Autodesk Inventor part; units mm, degrees
ref_plane "YZ Plane" through (0, 0, 0) normal (1, 0, 0) x (0, 1, 0)
ref_plane "XZ Plane" through (0, 0, 0) normal (0, 1, 0) x (-1, 0, 0)
ref_plane "XY Plane" through (0, 0, 0) normal (0, 0, 1) x (1, 0, 0)
sketch "スケッチ1" plane through (0, 0, 0) normal (0, 0, 1) x (1, 0, 0)
  circle A0 centre (0, 0) radius 23.5
  circle A1 centre (0, 0) radius 4
  dimension "d0" = 47
  dimension "d1" = 8
extrude "押し出し1" add sketch "スケッチ1" along normal blind 2
sketch "スケッチ2" plane through (0, 0, 2) normal (0, 0, 1) x (1, 0, 0)
  circle A0 centre (0, 0) radius 6.5 construction
  circle A1 centre (-6.5, 0) radius 1.75
  circle A2 centre (6.5, 0) radius 1.75
  dimension "d4" = 13
  dimension "d5" = 3.5
extrude "押し出し2" cut sketch "スケッチ2" against normal blind 2
chamfer "面取り1" distance 1.6 angle 45 2 edges at (-8.25, 0, 2) (4.75, 0, 2)
properties part number "SlitDiscSupport1"
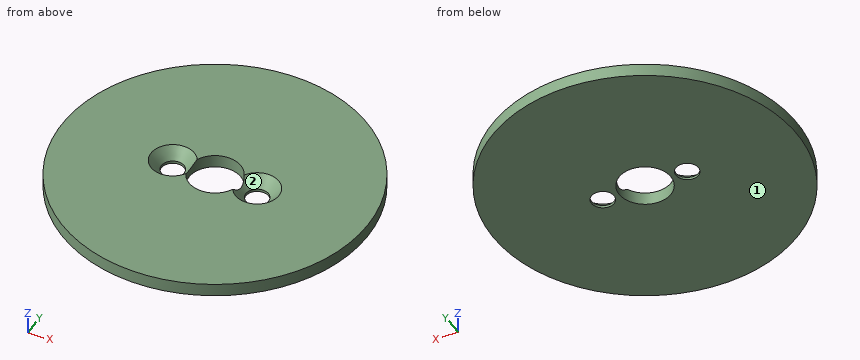
Part model, mm, in its own coordinate system. Face numbers are marked on the shaded views. Round coordinates to 2 decimals unless told otherwise and drop trailing zeros. Loops run counter-clockwise (first coordinate to the right, second up) from the corner with the lowest first, then second, coordinate; pieces in that order, holes last.
Item 1: Cut at B-B, the plane x = 0. Give the cut face in (y, z), then the cut area to 3 significant figures.
Item 2: Mould opens along X. For the marked faces 1 and 2 say: +X half, -X half, draft (parallel to the pull), parting line (faces both ways), or undercut.
Item 3: Drop flat-ended pins along their axis: P1, Ø5, axis at x = 0, y = 0, coming from the -Z side; P2, Ø5.5, axis at x = -6.5, y = 0, coming from the +Z side. Give the stop position or say it passes through.
Item 4: Cut at D-D, the plane x = -6.5. Give the cut face in (y, z).
Item 5: Cut at C-C, the plane z = 0.75. Give the cut face in (x, y).
Item 6: Drill centre lines: line 1 (Y direction, x = 0, z = 1.05); line 2 (Y direction, x = 5.5, z = 0.65); line 3 (X direction, y = -2.5, z = 0.2). Where is each one in solid material? Low to high.
Item 7: Cut at A-A, the plane y = 0. Give the cut face in (x, z), then the cut area to 3 significant figures.
A:
1. outline: (-23.5, 0) - (-4, 0) - (-4, 2) - (-23.5, 2) - close; (4, 0) - (23.5, 0) - (23.5, 2) - (4, 2) - close
1. area: 78.0 mm2
2. face 1: draft
2. face 2: undercut
3. P1: passes through
3. P2: stops at z = 1.4
4. outline: (-22.58, 0) - (-1.75, 0) - (-1.75, 0.4) - (-3.35, 2) - (-22.58, 2) - close; (1.75, 0) - (22.58, 0) - (22.58, 2) - (3.35, 2) - (1.75, 0.4) - close
5. outline: circle Ø47 at (0, 0); hole circle Ø4.2 at (-6.5, 0); hole circle Ø8 at (0, 0); hole circle Ø4.2 at (6.5, 0)
6. line 1: y = -23.5 to -4, 4 to 23.5
6. line 2: y = -22.85 to -1.73, 1.73 to 22.85
6. line 3: x = -23.37 to -3.12, 3.12 to 23.37
7. outline: (-23.5, 0) - (-8.25, 0) - (-8.25, 0.4) - (-9.85, 2) - (-23.5, 2) - close; (-4.75, 0) - (-4, 0) - (-4, 1.15) - (-4.75, 0.4) - close; (4, 0) - (4.75, 0) - (4.75, 0.4) - (4, 1.15) - close; (8.25, 0) - (23.5, 0) - (23.5, 2) - (9.85, 2) - (8.25, 0.4) - close
7. area: 59.6 mm2
